Geometry: final body of the model. Coordinates: model frame, mm. A direction names the side the tool comes from. Round coordinates to 2 decimals unless told otherwise and drop trailing zeros. Write each loop counter-clockwise with the first axis right and the second up, starting at its lowest first coordinate (ties: lowest second). Pieces come first, ordered by that corner, then holes. Notation, with made-up numbers: (50.25, 30.5) - (59.25, 30.5) arc R21 ccw to (59.25, 64.5) - close; hole circle Ø11 at (-37.75, 31). An arc over 180 degrees is marked (long way). Write each question's results on one line, items separated by ' | '.
from build123d import *

# Parameters (mm, degrees)
F1_DEPTH = 20
F2_R     = 2
F3_R     = 1
F4_R     = 5


with BuildPart() as f1:
    # F0 (on Top) → F1 (new body)
    with BuildSketch(Plane.XY):
        Polygon((0, 16), (0, 0), (2, 0), (2, 14), (50, 14), (50, 16), (2, 18), (-10, 17), (-10, 16), align=None)
    extrude(amount=F1_DEPTH)

    # F2
    f2_edges = [f1.edges().sort_by_distance(p)[0] for p in [
        (50, 16, 10),
        (2, 14, 10),
    ]]
    fillet(f2_edges, radius=F2_R)

    # F3
    f3_edges = [f1.edges().sort_by_distance(p)[0] for p in [
        (-10, 17, 10),
    ]]
    fillet(f3_edges, radius=F3_R)

    # F4
    f4_edges = [f1.edges().sort_by_distance(p)[0] for p in [
        (2, 18, 10),
    ]]
    fillet(f4_edges, radius=F4_R)


solid = f1.part
Q1. Section query A-A, the plane z = 4.75. Return loops of the section in (x, y).
Answer block:
outline: (-10, 16) - (0, 16) - (0, 0) - (2, 0) - (2, 12) arc R2 cw to (4, 14) - (50, 14) - (50, 14.08) arc R2 ccw to (48.08, 16.08) - (2.31, 17.99) arc R5 ccw to (1.69, 17.97) - (-9.08, 17.08) arc R1 ccw to (-10, 16.08) - close
Q2. Section query C-C, the plane x = -1. Return loops of the section in (y, z).
Answer block:
outline: (16, 0) - (17.75, 0) - (17.75, 20) - (16, 20) - close
Q3. Section query B-B, the plane y = 8.25. Return loops of the section in (x, z), plus the area to 3 significant figures.
Answer block:
outline: (0, 0) - (2, 0) - (2, 20) - (0, 20) - close | area: 40.0 mm2
Q4. Ray query, line 1 along X through (y, z) = (1.75, 17); line 2 along Y through (x, z) = (-7.5, 12); line 3 along Y through (x, z) = (31, 12.75). Return the intervals inside material, ascending.
Answer block:
line 1: 0 to 2 | line 2: 16 to 17.21 | line 3: 14 to 16.79
Q5. Pin query (flat end, axial travel): pin 1 (10 mm diameter, centred on x = 10, z = 4, fed in from -Y); pin 2 (3 mm diameter, centred on y = 8.5, z = 12, fed in from +X); pin 3 (8 mm diameter, centred on y = 5.5, z = 3.5, fed in from -X). Return the tip coordinate at first contact, or that it passes through.
Answer block:
pin 1: y = 14 | pin 2: x = 2 | pin 3: x = 0
Q6. Access query for faces 1 (the flat face through (0, 8, 10)), 2 (the flat face through (-3.62, 17.53, 9.86)), 3 (the flat face through (2, 6, 10)). Directions: +Z, -Z, +X, -X, +Y, -Y. A direction counts if a zero-diameter tool reaches every point of the face in a straight line with its end or side. Return the directions, or none.
Answer block:
face 1: +Z, -Z, -X, -Y | face 2: +Z, -Z, -X, +Y | face 3: +Z, -Z, +X, -Y
